Read the model definition and answer for the solid it produces. Units are mm, in the model's axes. A direction names the side the tool comes from. Coordinates: 2 decimals unless noted, no trailing zeros. Order: outer loops, then holes, each group sorted by start corner. A loop starts at its lowest first (then second) coordinate and runs counter-clockwise, first axis right, second up. Notation, with made-up numbers: M 64,-24.75 L 120,-24.75 A31 cw 120,5.25 Z; hole C -27.5,22 d2. An arc over 180 degrees is marked long. Use a Markdown table: item, result. Add a question column.
1) For faces 5 (the face through (26, 11, -36)), 6 (the face through (0, 1, -11)), 7 (the face through (25.141, 11.736, -20.203)), determine the directions among +Z, -Z, +X, -X, +Y, -Y from which every point of the face is accessible in a straight line to the end or side of a thin tool.
2) The mould has two halves that part along Z. Classify faces 1 (the face through (35, 11, 14)), 2 (the face through (25.43, 11.15, -48.4)), 3 (the face through (0, 11, 47)), 4 (the face through (0, 1, -39)): released by +Z, released by -Z, zero draft, split by the parting line, or undercut.
3) Find section A-A on x = 23. Write down the section's boundary in (y, z), plus the area to 3 significant figures.
4) Find section D-D on z = 40.5. Write down the section's boundary in (x, y), plus the area to 3 significant figures.
5) Find the intervals of material crossed by probe 1 along X at (y, z) = (10.5, 23.5); probe 2 along Z at (x, y) = (-14, 6.5); probe 3 along X at (y, z) = (1.25, -4.5), in increasing order. Write a range as [from, to].
6) Each of these flat-tipped pins is pushed along its axis until it touches: pin 1 Ø11 at (y, z) = (15.5, -35) entering from -X; pin 2 Ø6 at (x, y) = (26, 9) entering from -Z; pin 3 Ø10 at (x, z) = (-27, 24.5) entering from +Y; pin 4 Ø10 at (y, z) = (6, -29) entering from -X. Where does it stop, or does it pass through?
7) Find section B-B on z = 10. Write down the section's boundary in (x, y), plus the area to 3 significant figures.
from build123d import *

# Parameters (mm, degrees)
SKETCH1_W               = 50
SKETCH1_H               = 50
SKETCH1_W_2             = 48
SKETCH1_H_2             = 8
BOSS_EXTRUDE1_DEPTH     = 2
FILLET1_R               = 4
FILLET2_R               = 2
BOSS_EXTRUDE2_START     = 20
BOSS_EXTRUDE2_DEPTH     = 20
CUT_EXTRUDE1_DEPTH      = 65.109281699
CUT_EXTRUDE1_DEPTH_BACK = 65.109281699


with BuildPart() as part:
    # Sketch1 → Boss-Extrude1 (new body)
    with BuildSketch(Plane(origin=(0, 0, 0), x_dir=(1, 0, 0), z_dir=(0, 1, 0))):
        Polygon((26, 49), (-26, 49), (-26, 21), (-35, 21), (-35, -49), (35, -49), (35, 21), (26, 21), align=None)
        with Locations((0, -14)):
            Rectangle(SKETCH1_W, SKETCH1_H, mode=Mode.SUBTRACT)
        with Locations((0, 25)):
            Rectangle(SKETCH1_W_2, SKETCH1_H_2, mode=Mode.SUBTRACT)
        with Locations((0, 43)):
            Rectangle(SKETCH1_W_2, SKETCH1_H_2, mode=Mode.SUBTRACT)
    extrude(amount=BOSS_EXTRUDE1_DEPTH)

    # Fillet1
    fillet1_edges = [part.edges().sort_by_distance(p)[0] for p in [
        (35, 1, -21),
        (35, 1, 49),
        (-35, 1, 49),
        (-35, 1, -21),
        (-26, 1, -21),
        (26, 1, -21),
    ]]
    fillet(fillet1_edges, radius=FILLET1_R)

    # Fillet2
    fillet2_edges = [part.edges().sort_by_distance(p)[0] for p in [
        (-26, 1, -49),
        (26, 1, -49),
    ]]
    fillet(fillet2_edges, radius=FILLET2_R)

    # Sketch4 → Boss-Extrude2 (add)
    with BuildSketch(Plane(origin=(0, 2, 0), x_dir=(1, 0, 0), z_dir=(0, 1, 0)).offset(BOSS_EXTRUDE2_START)):
        with BuildLine():
            Line((-31, -49), (31, -49))
            ThreePointArc((31, -49), (33.828427125, -47.828427125), (35, -45))
            Line((35, -45), (35, 17))
            ThreePointArc((35, 17), (33.828427125, 19.828427125), (31, 21))
            Line((31, 21), (30, 21))
            ThreePointArc((30, 21), (27.171572875, 22.171572875), (26, 25))
            Line((26, 25), (26, 47))
            ThreePointArc((26, 47), (25.414213562, 48.414213562), (24, 49))
            Line((24, 49), (-24, 49))
            ThreePointArc((-24, 49), (-25.414213562, 48.414213562), (-26, 47))
            Line((-26, 47), (-26, 25))
            ThreePointArc((-26, 25), (-27.171572875, 22.171572875), (-30, 21))
            Line((-30, 21), (-31, 21))
            ThreePointArc((-31, 21), (-33.828427125, 19.828427125), (-35, 17))
            Line((-35, 17), (-35, -45))
            ThreePointArc((-35, -45), (-33.828427125, -47.828427125), (-31, -49))
        make_face()
        with BuildLine():
            Line((-29, 19), (-28, 19))
            ThreePointArc((-28, 19), (-25.171572875, 20.171572875), (-24, 23))
            Line((-24, 23), (-24, 47))
            Line((-24, 47), (24, 47))
            Line((24, 47), (24, 23))
            ThreePointArc((24, 23), (25.171572875, 20.171572875), (28, 19))
            Line((28, 19), (29, 19))
            ThreePointArc((29, 19), (31.828427125, 17.828427125), (33, 15))
            Line((33, 15), (33, -43))
            ThreePointArc((33, -43), (31.828427125, -45.828427125), (29, -47))
            Line((29, -47), (-29, -47))
            ThreePointArc((-29, -47), (-31.828427125, -45.828427125), (-33, -43))
            Line((-33, -43), (-33, 15))
            ThreePointArc((-33, 15), (-31.828427125, 17.828427125), (-29, 19))
        make_face(mode=Mode.SUBTRACT)
    extrude(amount=-BOSS_EXTRUDE2_DEPTH)

    # Sketch6 → Cut-Extrude1 (cut, two sides: drawn at the far end of the back side and taken through both)
    with BuildSketch(Plane(origin=(0, 0, 0), x_dir=(0, 0, -1), z_dir=(1, 0, 0)).offset(-CUT_EXTRUDE1_DEPTH_BACK)):
        Polygon((-49, 22), (-49, 19), (49, 22), align=None)
    extrude(amount=CUT_EXTRUDE1_DEPTH + CUT_EXTRUDE1_DEPTH_BACK, mode=Mode.SUBTRACT)


solid = part.part
Check result:
| question | item | result |
|---|---|---|
| 1 | face 5 | -Z, +X, +Y, -Y |
| 1 | face 6 | +Y, -Y |
| 1 | face 7 | +Y |
| 2 | face 1 | zero draft |
| 2 | face 2 | released by -Z |
| 2 | face 3 | undercut |
| 2 | face 4 | undercut |
| 3 | outline | M 0,-49 L 22,-49 L 21.94,-47 L 0,-47 Z; M 0,-39 L 2,-39 L 2,-29 L 0,-29 Z; M 0,-21 L 2,-21 L 2,-11 L 0,-11 Z; M 0,39 L 2,39 L 2,47 L 19.06,47 L 19,49 L 0,49 Z |
| 3 | area | 138 mm2 |
| 4 | outline | M -35,0 L 35,0 L 35,19.26 L 33,19.26 L 33,2 L -33,2 L -33,19.26 L -35,19.26 Z |
| 4 | area | 209 mm2 |
| 5 | probe 1 | x = [-35, -33], [33, 35] |
| 5 | probe 2 | z = [-49, -47], [47, 49] |
| 5 | probe 3 | x = [-35, -25], [25, 35] |
| 6 | pin 1 | stops at x = -26 |
| 6 | pin 2 | stops at z = -49 |
| 6 | pin 3 | stops at y = 2 |
| 6 | pin 4 | stops at x = -26.13 |
| 7 | outline | M -35,0 L -25,0 L -25,2 L -33,2 L -33,20.19 L -35,20.19 Z; M 25,0 L 35,0 L 35,20.19 L 33,20.19 L 33,2 L 25,2 Z |
| 7 | area | 113 mm2 |
